Geometry check sheet. Reference: the model listing, model coordinates, mm. A direction names the side the tool comes from. Give positions to 0.01 mm unless a question says otherwise; leave off trailing zeros. Loops run counter-clockwise (first coordinate to the right, second up) from the corner with the lowest first, then second, coordinate; pieces in that order, holes last. Notation, with made-up numbers: (-37, -17) -> (19, -17) arc R17 cw to (19, -5) -> close; hole circle Ø6 at (58, -8). An arc over 180 degrees is marked (long way). Answer as a JSON object with one key per item and string values.
Autodesk Inventor part; units mm, degrees
ref_plane "Work Plane2" through (3.35, 0, 0) normal (0, 0, -1) x (1, 0, 0)
ref_plane "YZ Plane" through (0, 0, 0) normal (1, 0, 0) x (0, 1, 0)
ref_plane "XZ Plane" through (0, 0, 0) normal (0, 1, 0) x (-1, 0, 0)
sketch "Sketch1" plane through (0, 0, 0) normal (0, 0, 1) x (1, 0, 0)
  line L0 (2.6, 0) -> (25, 0)
  line L1 (25, 0) -> (25, 2)
  line L2 (25, 2) -> (4.1, 2)
  line L3 (4.1, 2) -> (3.6706, 1.7853)
  line L4 (3.6706, 1.7853) -> (2.7, 1.7853)
  line L5 (0, 4.2) -> (0, 2.3)
  line L6 (0, 2.3) -> (1.8738, 1.3657)
  line L7 (1.8738, 1.3657) -> (2.6, 0)
  line L8 (-5, 0) -> (30, 0)
  line L9 (0, -0.84) -> (0, 5.04)
  line L10 (0, 4.2) -> (0.2853, 4.2)
  line L11 (0.2853, 4.2) -> (2.7, 1.7853)
  line L12 (4.1, 2) -> (2.4853, 2) construction
  dimension "d1" = 20.9
  dimension "d2" = 4
  dimension "d3" = 3.5706
  dimension "d4" = 4.6
  dimension "d5" = 26.5
  dimension "d6" = 62
  dimension "d7" = 2.6
  dimension "d8" = 0.4294
  dimension "d12" = 8.4
  dimension "d13" = 45
  dimension "d15" = 25
  dimension "d24" = 2.7
revolve "Body" add sketch "Sketch1" angle 360 about axis through (2.6, 0, 0) along (1, 0, 0) contours L7 L6 L5 L10 L11 L4 L3 L2 L1 L0
sketch "Sketch2" plane through (0, 0, 0) normal (-1, 0, 0) x (0, 0, 1)
  line L0 (0, 2.3) -> (0, 0) construction
  line L1 (0, 0) -> (2.3, 0) construction
  arc A0 (0.69, 0) -> (0, 0.69) centre (0, 0) ccw construction
  arc A1 (0.805, 0) -> (0, 0.805) centre (0, 0) ccw construction
  arc A2 (2.2762, 0.33) -> (0.33, 2.2762) centre (0, 0) ccw
  line L2 (0, 0) -> (1.6263, 1.6263) construction
  line L3 (0.33, 2.2762) -> (0.3941, 0.7019)
  line L4 (2.2762, 0.33) -> (0.7019, 0.3941)
  arc A3 (0.33, 2.2762) -> (0, 2.3) centre (0, 0) ccw
  arc A4 (2.3, 0) -> (2.2762, 0.33) centre (0, 0) ccw
  line L5 (0, -5.88) -> (0, 5.88)
  line L6 (-5.88, 0) -> (5.88, 0)
  arc A5 (0.33, -2.2762) -> (2.2762, -0.33) centre (0, 0) ccw
  line L7 (0.33, -2.2762) -> (0.3941, -0.7019)
  line L8 (2.2762, -0.33) -> (0.7019, -0.3941)
  arc A6 (0, -2.3) -> (0.33, -2.2762) centre (0, 0) ccw
  arc A7 (2.2762, -0.33) -> (2.3, 0) centre (0, 0) ccw
  arc A8 (-0.33, 2.2762) -> (-2.2762, 0.33) centre (0, 0) ccw
  line L9 (-0.33, 2.2762) -> (-0.3941, 0.7019)
  line L10 (-2.2762, 0.33) -> (-0.7019, 0.3941)
  arc A9 (0, 2.3) -> (-0.33, 2.2762) centre (0, 0) ccw
  arc A10 (-2.2762, 0.33) -> (-2.3, 0) centre (0, 0) ccw
  arc A11 (-0.33, -2.2762) -> (0, -2.3) centre (0, 0) ccw
  arc A12 (-2.2762, -0.33) -> (-0.33, -2.2762) centre (0, 0) ccw
  arc A13 (-2.3, 0) -> (-2.2762, -0.33) centre (0, 0) ccw
  line L11 (-2.2762, -0.33) -> (-0.7019, -0.3941)
  line L12 (-0.33, -2.2762) -> (-0.3941, -0.7019)
  arc A14 (0.3941, 0.7019) -> (0.7019, 0.3941) centre (0.715, 0.715) ccw
  arc A15 (0.7019, -0.3941) -> (0.3941, -0.7019) centre (0.715, -0.715) ccw
  arc A16 (-0.7019, 0.3941) -> (-0.3941, 0.7019) centre (-0.715, 0.715) ccw
  arc A17 (-0.3941, -0.7019) -> (-0.7019, -0.3941) centre (-0.715, -0.715) ccw
  point P0 (1.6263, -1.6263)
  point P1 (-1.6263, 1.6263)
  point P2 (-1.6263, -1.6263)
  dimension "d17" = 1.38
  dimension "d18" = 1.61
  dimension "d19" = 4.6
  dimension "d20" = 45
  dimension "d21" = 0.33
extrude "Slot" add sketch "Sketch2" against normal up to next draft 5 contours L4 A14 L3 A2 | A5 L7 A15 L8 | L9 A16 L10 A8 | A12 L11 A17 L12
fillet "Fillet1" radius 0.132 4 edges at (0, 2.3, 0) (0, 0, -2.3) (0, -2.3, 0) (0, 0, 2.3)
thread "Thread"
chamfer "Chamfer1" distance 0.4294 distance2 0.2147 1 edges at (25, -2, 0) measured on face at (25, -0.9099, 0.3408)
ref_plane "Work Plane2" through (3.35, 0, 0) normal (0, 0, -1) x (1, 0, 0)
equation "\"d1\" = GEL"
equation "\"d2\" = GD"
equation "\"d3\" = BDM"
equation "\"d4\" = SDM"
equation "\"d7\" = INTI"
equation "\"d8\" = GAL"
equation "\"d12\" = KOD"
equation "\"d13\" = 0.5 * SEWI"
equation "\"d15\" = NLG"
equation "\"d24\" = KOH"
equation "\"d17\" = 0.3 * SDM"
equation "\"d18\" = 0.35 * SDM"
equation "\"d19\" = SDM"
equation "\"d21\" = 0.5 * SBR"
equation "\"d23\" = 0.2 * SBR"
equation "\"d10\" = GEL"
equation "\"d25\" = -0.5 * SPD + 0.5 * GD"
equation "\"d26\" = 0.5 * GAL"
equation "\"NLG\" = 25"
equation "\"GEL\" = 20.9"
equation "\"GAL\" = 0.61345 * PTC"
equation "\"SPD\" = NND - 1.2269 * PTC"
equation "\"KOD\" = 8.4"
equation "\"KOH\" = 2.7"
equation "\"SBR\" = 0.66"
equation "\"INTI\" = 2.6"
equation "\"SDM\" = 4.6"
equation "\"GD\" = NND"
equation "\"BDM\" = NND - GAL"
equation "\"SEWI\" = 90deg"
equation "\"d9\" = SDM"
equation "\"GUL\" = 0.61345 * PTC"
equation "\"TOA\" = 30deg"
equation "\"EPV\" = 4.7"
equation "\"THREADDIA\" = 4"
equation "\"PTC\" = 0.7"
equation "\"NND\" = 4"
equation "\"GD1\" = THREADDIA - 1.2269 * PTC"
properties part number "ISO 7046-1 - M4 x 25 - 4.8 - H" material "Steel"
1) Material ranges on line 1 along X through (y, z) = (-2.25, -3.5); line 2 along Z through (x, y) = (17, 0); line 3 along X through (y, z) = (0, 3.5), recorded low to high. Write a range as from..to.
Geometry check:
{"line 1": "x = 0..0.32", "line 2": "z = -2..2", "line 3": "x = 0..0.99"}
2) Tool access check on faces 4 (the face through (14, 0, 2)), 5 (the face through (1, 0, 1.8)), 6 (the face through (3.179, -0.387, 1.743)). Record the directions out of +Z, -Z, +X, -X, +Y, -Y that give a thin tool (end or side, any length) a straight path to the whole face; none if there is none.
Geometry check:
{"face 4": "+X", "face 5": "-X", "face 6": "none"}
3) Depth check by flat-ended pin: P1, Ø1.5, axis at x = 15.5, z = -0.5, coming from the +Y side; P2, Ø4, axis at x = 4.5, y = -1.5, coming from the +Z side; P3, Ø5, axis at x = 15, z = 1.5, coming from the -Y side; P4, Ø1.5, axis at y = -0.5, z = 0.5, coming from the -X side. Enter the tip coordinate at first touch or a pass-through.
Geometry check:
{"P1": "stops at y = 2", "P2": "stops at z = 2", "P3": "stops at y = -2", "P4": "stops at x = 0"}
4) Draft check along Z on faces 1 (the face through (2.55, 0.89, 1.72)), 2 (the face through (0.846, -1.355, -0.293)), 3 (the face through (25, 0, 0)). Enter one of: pulls with the +Z half, pulls with the -Z half, needs draft (parallel to the pull), parting line crosses it, or undercut.
Geometry check:
{"face 1": "parting line crosses it", "face 2": "undercut", "face 3": "needs draft"}
5) Section check A-A on x = 6.25. Record the cut outline in (y, z), plus the area to 3 significant figures.
Geometry check:
{"outline": "circle Ø4 at (0, 0)", "area": "12.6 mm2"}
